Design review of the part shown in the three views and the two pictorial views. Dimensions are in mm from the part's minimum x, y and z. Coordinates: 2 decimals unless noted, no trailing zeros. Loops run counter-clockwise (first coordinate to the right, second up) from the corner with the lowest first, then second, coordinate; pieces in that order, holes last. Notation, with made-up numbers: M 2.25,67.25 L 16.25,67.25 A35 ccw 16.25,99.25 Z; hole C 45.5,77.5 d5. An arc over 180 degrees is marked long. Put each result on its own line as item: value. Start each with the question number.
(1) Clearance check with a flat-ended pin moving along its axis: pin 1 (5 mm diameter, centred on x = 39, y = 22, fed in from +Z). State where the tip first meets the part, or that it passes through.
(2) The part is to be moulded in two halves that separate along X. For the marked faces 1, 2 and 3, say which applies: +X half, -X half, draft (parallel to the pull), parting line (faces both ways), or undercut.
(3) Take a section at C-C, the plane x = 19. Give the boundary of the cut face in (y, z), then the cut area to 3 significant figures.
(4) Take a section at A-A, the plane z = 102. Give the boundary of the cut face in (x, y), then the cut area to 3 significant figures.
(5) For probe 1 along X at (y, z) = (9, 107.5); probe 2 along Z at (x, y) = (29.5, 40.5); probe 3 along Z at (x, y) = (42.5, 9), list the stretches that pass through material, from the lowest coordinate up. Write a range as [from, to].
(6) Take a section at B-B, the plane y = 41.5. Give the boundary of the cut face in (x, z) (3 decimals).
(7) Take a section at D-D, the plane x = 41. Give the boundary of the cut face in (y, z), then the cut area to 3 significant figures.
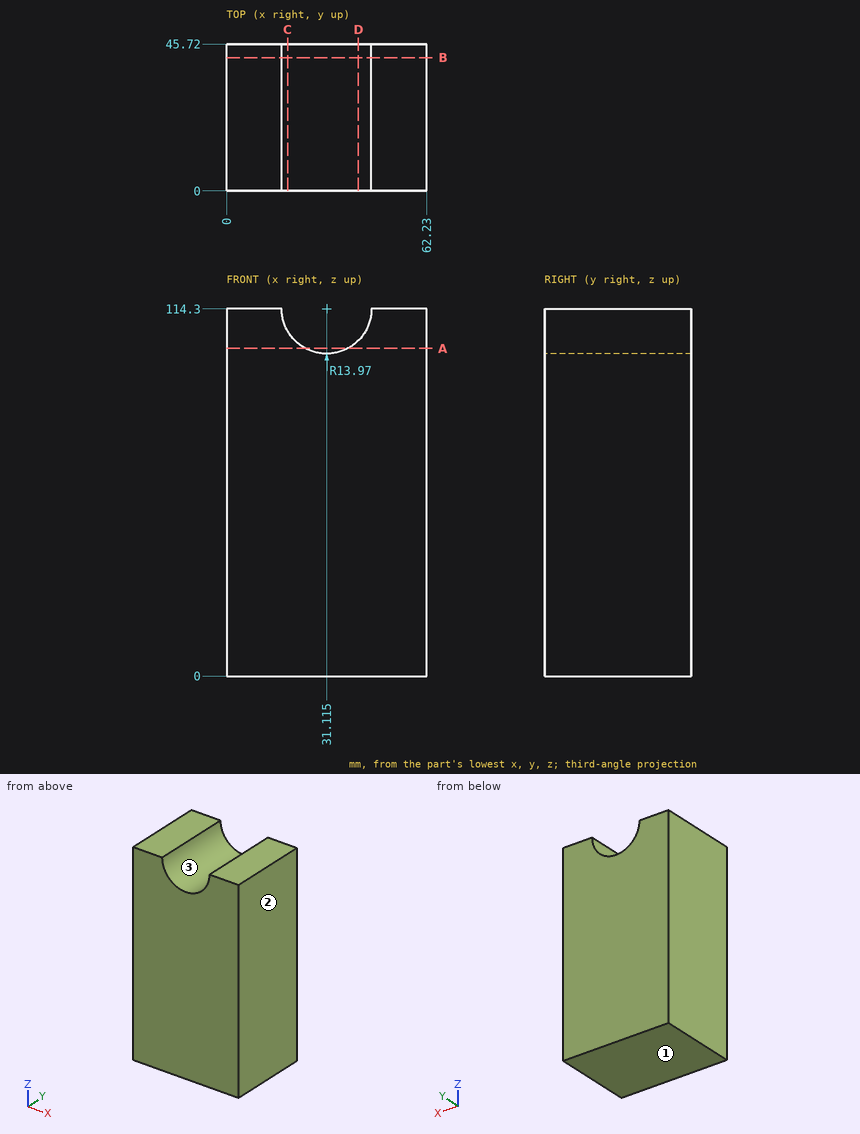
Computed values:
1. pin 1: stops at z = 104.96
2. face 1: draft
2. face 2: +X half
2. face 3: undercut
3. outline: M 0,0 L 45.72,0 L 45.72,107.34 L 0,107.34 Z
3. area: 4,910 mm^2
4. outline: M 0,0 L 24.49,0 L 24.49,45.72 L 0,45.72 Z; M 37.74,0 L 62.23,0 L 62.23,45.72 L 37.74,45.72 Z
4. area: 2,240 mm^2
5. probe 1: x = [0, 18.91], [43.32, 62.23]
5. probe 2: z = [0, 100.42]
5. probe 3: z = [0, 106.2]
6. outline: M 0,0 L 62.23,0 L 62.23,114.3 L 45.085,114.3 A13.97 cw 17.145,114.3 L 0,114.3 Z
7. outline: M 0,0 L 45.72,0 L 45.72,104.43 L 0,104.43 Z
7. area: 4,770 mm^2
